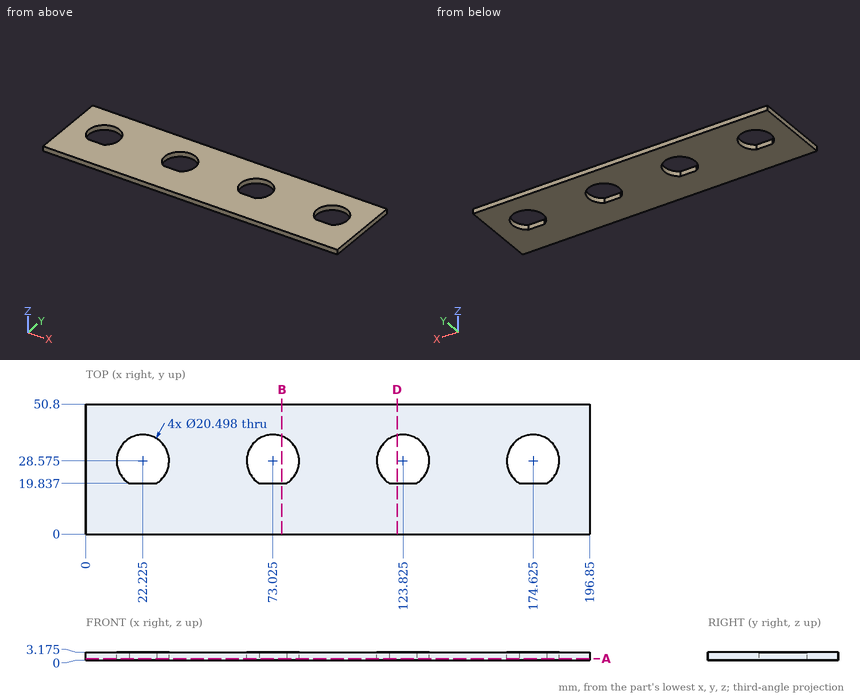
Source: three-view drawing plus pictorial views. Frame: mm from the lowest corner of the part. Give positions to 0.01 mm unless a question says otherwise; leave off trailing zeros. Order: outer loops, then holes, each group sorted by start corner. A loop starts at its lowest first (then second) coordinate and runs counter-clockwise, first axis right, second up. Notation, with made-up numbers: (-10.75, 52.25) - (28.25, 52.25) arc R21 cw to (28.25, 59.25) - close; hole circle Ø8 at (83, -20). An arc over 180 degrees is marked (long way). Put each result on its own line as item: value.
Item 1: Section query A-A, the plane z = 0.6. Count the separate pieces of the cut face and the enclosed holes in it, then the cut area to 3 significant figures.
Found:
separate pieces: 1
enclosed holes: 4
area: 8,720 mm^2
Item 2: Section query B-B, the plane x = 76.5. Return loops of the section in (y, z) (1 decimal), then the cut area to 3 significant figures.
Found:
outline: (0, 0) - (19.8, 0) - (19.8, 3.2) - (0, 3.2) - close; (38.2, 0) - (50.8, 0) - (50.8, 3.2) - (38.2, 3.2) - close
area: 103 mm^2
Item 3: Section query D-D, the plane x = 121.5. Return loops of the section in (y, z) (1 decimal).
Found:
outline: (0, 0) - (19.8, 0) - (19.8, 3.2) - (0, 3.2) - close; (38.6, 0) - (50.8, 0) - (50.8, 3.2) - (38.6, 3.2) - close
Item 4: Ray query, L1, parallel to X at y = 36, z = 2.9; L2, parallel to X at y = 34.5, z = 1.3; L3, parallel to Y at x = 72.5, z = 1.7. Return the intervals inside material, ascending. Write a range as from..to.
Found:
L1: x = 0..15.16, 29.29..65.96, 80.09..116.76, 130.89..167.56, 181.69..196.85
L2: x = 0..13.86, 30.59..64.66, 81.39..115.46, 132.19..166.26, 182.99..196.85
L3: y = 0..19.84, 38.81..50.8
